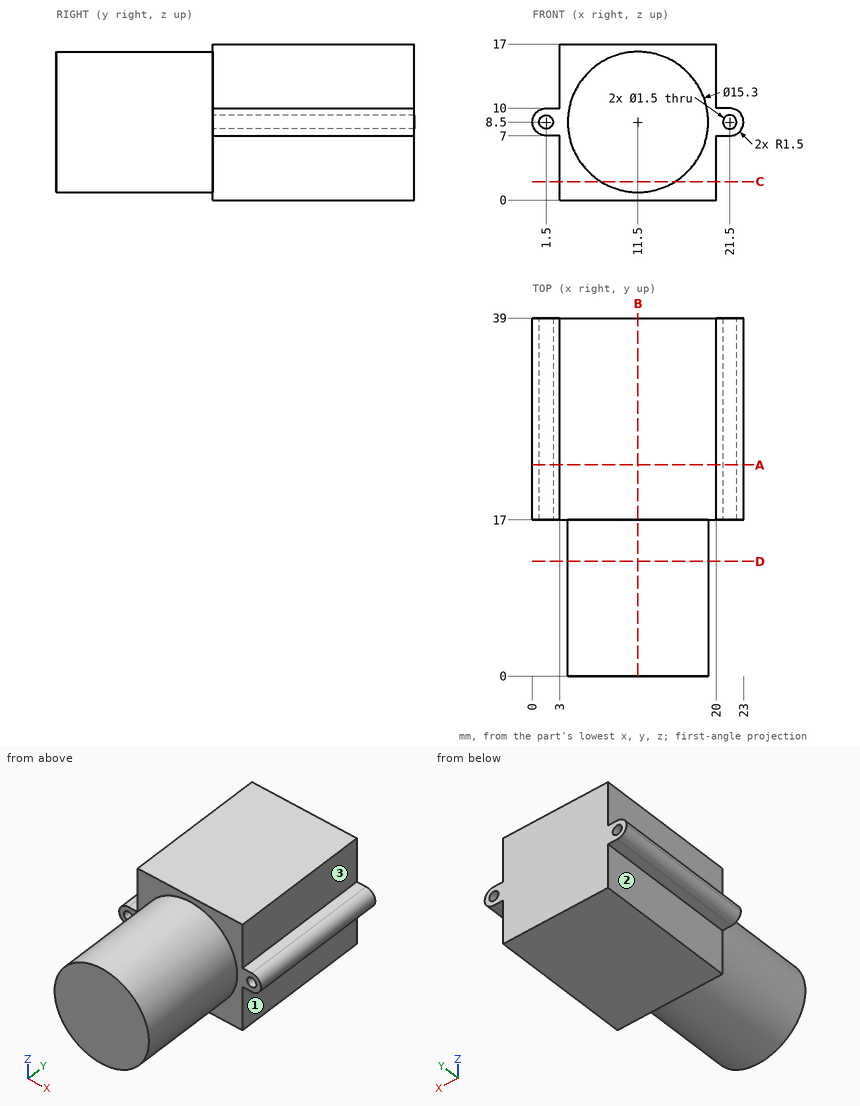
Drawing for the job (mm, zero at the part's lowest x, y, z). A direction names the side the tool comes from. Coordinates: 2 decimals unless noted, no trailing zeros. Write each loop counter-clockwise with the first axis right and the second up, starting at its lowest first coordinate (ties: lowest second). Pieces come first, ordered by that corner, then holes. Notation, with made-up numbers: (41, 59.25) - (50, 59.25) arc R8 cw to (50, 67.25) - close; hole circle Ø11 at (-4.5, 38). An arc over 180 degrees is marked (long way). Write each question's results on one line, items separated by ' | '. Start each with the question number.
1) Cut at A-A (y = 23). Write the cut outline in (x, z).
2) Flat gauge pins, fed straight in: P1, Ø1.7, axis at x = 1.5, z = 8.5, coming from the +Y side; P2, Ø5.5, axis at y = 31.5, z = 2, coming from the +X side; P3, Ø1.4, axis at x = 21.5, z = 8.5, coming from the -Y side; P4, Ø3.5, axis at y = 26.5, z = 14, coming from the -X side. Where does each tip first touch, or does it go through?
3) 3-axis set-ups, long thin cutter, end or side, ignore diameter. For the marked faces 1, 2 and 3: which of +Z, -Z, +X, -X, +Y, -Y reach the whole face in a straight line?
4) Cut at D-D (y = 12.5). Write the cut outline in (x, z), then the cut area to 3 significant figures.
5) Probe line 1 along Z through (x, y) = (21.5, 22.25); line 2 along X through (y, z) = (28, 3.25); line 3 along Z through (x, y) = (11.75, 7.5). List the from-to ranges inside material, lowest first. Write a range as from..to.
6) Cut at B-B (x = 11.5). Write the cut outline in (y, z), then the cut area to 3 significant figures.
7) Cut at C-C (z = 2). Write the cut outline in (x, y), then the cut area to 3 significant figures.
Returned:
1) outline: (1.5, 7) - (3, 7) - (3, 0) - (20, 0) - (20, 7) - (21.5, 7) arc R1.5 ccw to (21.5, 10) - (20, 10) - (20, 17) - (3, 17) - (3, 10) - (1.5, 10) arc R1.5 ccw to start; hole circle Ø1.5 at (1.5, 8.5); hole circle Ø1.5 at (21.5, 8.5)
2) P1: y = 39 | P2: x = 20 | P3: through | P4: x = 3
3) face 1: -Z, +X, +Y, -Y | face 2: -Z, -X, +Y, -Y | face 3: +Z, +X, +Y, -Y
4) outline: circle Ø15.3 at (11.5, 8.5) | area: 184 mm^2
5) line 1: 7..7.75, 9.25..10 | line 2: 3..20 | line 3: 0.85..16.15
6) outline: (0, 0.85) - (17, 0.85) - (17, 0) - (39, 0) - (39, 17) - (17, 17) - (17, 16.15) - (0, 16.15) - close | area: 634 mm^2
7) outline: (3, 17) - (7.47, 17) - (7.47, 0) - (15.53, 0) - (15.53, 17) - (20, 17) - (20, 39) - (3, 39) - close | area: 511 mm^2
